Here's how the part is built. I have some questions about the finished solid (model axes, mm). A direction names the side the tool comes from. Round coordinates to 2 decimals unless told otherwise and drop trailing zeros. Loops run counter-clockwise (first coordinate to the right, second up) from the corner with the lowest first, then second, coordinate; pieces in that order, holes last. Notation, with made-up numbers: (85.5, 35) -> (117.5, 35) arc R24 ccw to (117.5, 59) -> close; hole circle Ø4 at (36, -21). An arc over 180 degrees is marked (long way). One line per item, written item: value. Start each with the question number.
```python
from build123d import *

# Parameters (mm, degrees)
SKETCH_W     = 45.5
SKETCH_H     = 20.5
PAD_DEPTH    = 2.4
SKETCH001_R  = 8
PAD001_DEPTH = 12
SKETCH002_R  = 6.4
POCKET_DEPTH = 5
PAD002_DEPTH = 4
SKETCH004_W  = 10.5
SKETCH004_H  = 2.8
PAD003_DEPTH = 4
SKETCH005_W  = 1
SKETCH005_H  = 1
PAD004_DEPTH = 2
SKETCH006_W  = 1
SKETCH006_H  = 1
PAD005_DEPTH = 7.5
FILLET_R     = 0.5
FILLET001_R  = 0.5
CHAMFER_SIZE = 0.35


with BuildPart() as part:
    # Sketch → Pad (new body)
    with BuildSketch(Plane.XZ):
        Rectangle(SKETCH_W, SKETCH_H)
    extrude(amount=PAD_DEPTH)

    # Sketch001 → Pad001 (new body)
    with BuildSketch(Plane.XZ.offset(2.4)):
        with Locations((-12.75, 0)):
            Circle(SKETCH001_R)
        with Locations((12.75, 0)):
            Circle(SKETCH001_R)
    extrude(amount=PAD001_DEPTH)

    # Sketch002 → Pocket (cut)
    with BuildSketch(Plane.XZ.offset(14.4)):
        with Locations((-12.75, 0)):
            Circle(SKETCH002_R)
        with Locations((12.75, 0)):
            Circle(SKETCH002_R)
    extrude(amount=-POCKET_DEPTH, mode=Mode.SUBTRACT)

    # Sketch003 → Pad002 (new body)
    with BuildSketch(Plane.XZ.offset(2.4)):
        with BuildLine():
            ThreePointArc((-4.2, 8.25), (-6, 6.45), (-4.2, 4.65))
            Line((-4.2, 4.65), (4.2, 4.65))
            ThreePointArc((4.2, 4.65), (6, 6.45), (4.2, 8.25))
            Line((-4.2, 8.25), (4.2, 8.25))
        make_face()
    extrude(amount=PAD002_DEPTH)

    # Sketch004 → Pad003 (new body)
    with BuildSketch(Plane(origin=(0, 0, 0), x_dir=(1, 0, 0), z_dir=(0, 1, 0))):
        with Locations((0, 6.85)):
            Rectangle(SKETCH004_W, SKETCH004_H)
    extrude(amount=PAD003_DEPTH)

    # Sketch005 → Pad004 (new body)
    with BuildSketch(Plane(origin=(0, 4, 0), x_dir=(1, 0, 0), z_dir=(0, 1, 0))):
        with Locations((-3.75, 6.85)):
            Rectangle(SKETCH005_W, SKETCH005_H)
        with Locations((-1.25, 6.85)):
            Rectangle(SKETCH005_W, SKETCH005_H)
        with Locations((1.25, 6.85)):
            Rectangle(SKETCH005_W, SKETCH005_H)
        with Locations((3.75, 6.85)):
            Rectangle(SKETCH005_W, SKETCH005_H)
    extrude(amount=PAD004_DEPTH)

    # Sketch006 → Pad005 (new body)
    with BuildSketch(Plane(origin=(0, 0, -7.35), x_dir=(1, 0, 0), z_dir=(0, 0, -1))):
        with Locations((-3.75, -5.5)):
            Rectangle(SKETCH006_W, SKETCH006_H)
        with Locations((-1.25, -5.5)):
            Rectangle(SKETCH006_W, SKETCH006_H)
        with Locations((1.25, -5.5)):
            Rectangle(SKETCH006_W, SKETCH006_H)
        with Locations((3.75, -5.5)):
            Rectangle(SKETCH006_W, SKETCH006_H)
    extrude(amount=PAD005_DEPTH)

    # Fillet
    fillet_edges = [part.edges().sort_by_distance(p)[0] for p in [
        (-3.75, 6, -6.35),
        (-1.25, 6, -6.35),
        (1.25, 6, -6.35),
        (3.75, 6, -6.35),
    ]]
    fillet(fillet_edges, radius=FILLET_R)

    # Fillet001
    fillet001_edges = [part.edges().sort_by_distance(p)[0] for p in [
        (3.75, 5, -7.35),
        (1.25, 5, -7.35),
        (-1.25, 5, -7.35),
        (-3.75, 5, -7.35),
    ]]
    fillet(fillet001_edges, radius=FILLET001_R)

    # Chamfer
    chamfer_edges = [part.edges().sort_by_distance(p)[0] for p in [
        (-3.75, 6, -14.85),
        (-4.25, 5.5, -14.85),
        (-3.75, 5, -14.85),
        (-3.25, 5.5, -14.85),
        (-1.25, 6, -14.85),
        (-1.75, 5.5, -14.85),
        (-1.25, 5, -14.85),
        (-0.75, 5.5, -14.85),
        (1.25, 6, -14.85),
        (0.75, 5.5, -14.85),
        (1.25, 5, -14.85),
        (1.75, 5.5, -14.85),
        (3.75, 6, -14.85),
        (3.25, 5.5, -14.85),
        (3.75, 5, -14.85),
        (4.25, 5.5, -14.85),
    ]]
    chamfer(chamfer_edges, length=CHAMFER_SIZE)


solid = part.part
```
Q1. Will these pins go through, and if not, where does the flat tip stop? P1, Ø1.2, axis at x = 1, y = -5, coming from the -Z side; P2, Ø1.1, axis at x = 1.5, y = 5, coming from the +Z side; P3, Ø1.1, axis at x = -4, y = 4.5, coming from the +Z side; P4, Ø3, axis at y = 1, z = -7, coming from the -X side.
Q2. If we mould it in two halves opening along Z, with no side actions, what happens to faces 6 (the flat face through (-4, 5, -6.35)), 7 (the flat face through (0, -6.4, 6)), 8 (the cylindrical face through (-6, -4.4, 6.5))? For each: released by +Z, released by -Z, zero draft, split by the parting line, or undercut.
Q3. I want a section at A-A on y = -12.5. Please give me the cut outline in (x, z).
Q4. I want a section at B-B on x = 12.75. Please give me the cut outline in (y, z), plus the area to 3 significant figures.
Q5. I want a section at C-C on z = 0. Please give me the cut outline in (x, y), plus the area to 3 significant figures.
Q6. If I drill on line 1 along Y through (x, z) = (4, -11.5); line 2 along Z through (x, y) = (12.75, -11.9); line 3 along Y through (x, z) = (12.5, 3), over which ranges is the centre line in solid material (lowest first)?
Q7. I want a section at D-D on y = 3. Please give me the cut outline in (x, z), plus the area to 3 significant figures.
Q8. Which directions (+Z, -Z, +X, -X, +Y, -Y) give clear straight access to the entire face, cutting with the end or side of a thin tool? Please do faces 1 (the flat face through (0, 4, -7)), 2 (the cylindrical face through (-19.144, -11.935, 0.281)), 3 (the flat face through (0, 2, -5.45)), 4 (the flat face through (-3.25, 5.5, -10.4)), 5 (the flat face through (0, -4, 4.65)).
Answers below:
1. P1: stops at z = 4.65
1. P2: stops at z = -6.35
1. P3: stops at z = -5.45
1. P4: stops at x = -22.75
2. face 6: released by +Z
2. face 7: zero draft
2. face 8: undercut
3. outline: circle Ø16 at (-12.75, 0); circle Ø16 at (12.75, 0); hole circle Ø12.8 at (-12.75, 0); hole circle Ø12.8 at (12.75, 0)
4. outline: (-14.4, -8) -> (-2.4, -8) -> (-2.4, -10.25) -> (0, -10.25) -> (0, 10.25) -> (-2.4, 10.25) -> (-2.4, 8) -> (-14.4, 8) -> (-14.4, 6.4) -> (-9.4, 6.4) -> (-9.4, -6.4) -> (-14.4, -6.4) -> close
4. area: 177 mm^2
5. outline: (-22.75, -2.4) -> (-20.75, -2.4) -> (-20.75, -14.4) -> (-19.15, -14.4) -> (-19.15, -9.4) -> (-6.35, -9.4) -> (-6.35, -14.4) -> (-4.75, -14.4) -> (-4.75, -2.4) -> (4.75, -2.4) -> (4.75, -14.4) -> (6.35, -14.4) -> (6.35, -9.4) -> (19.15, -9.4) -> (19.15, -14.4) -> (20.75, -14.4) -> (20.75, -2.4) -> (22.75, -2.4) -> (22.75, 0) -> (-22.75, 0) -> close
5. area: 365 mm^2
6. line 1: y = 5 to 6
6. line 2: z = -8 to -6.4, 6.4 to 8
6. line 3: y = -9.4 to 0
7. outline: (-5.25, -8.25) -> (5.25, -8.25) -> (5.25, -5.45) -> (-5.25, -5.45) -> close
7. area: 29.4 mm^2
8. face 1: none
8. face 2: -Y
8. face 3: +Z, +X, -X, +Y
8. face 4: +Z, -Z, +Y
8. face 5: -Z, -Y
